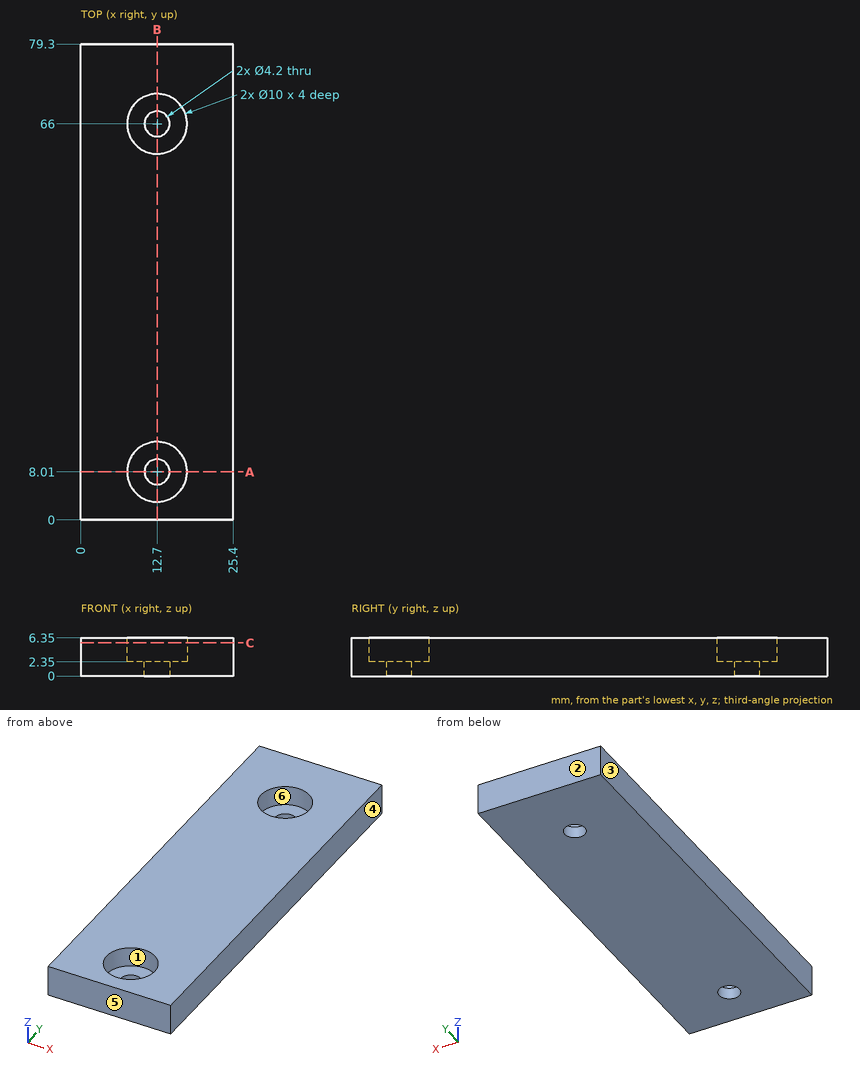
The drawing under review shows one solid part. Ordinate dimensions are in mm from its lowest x, y, z. A direction names the side the tool comes from. Coordinates: 2 decimals unless noted, no trailing zeros. Order: outer loops, then holes, each group sorted by start corner. A loop starts at its lowest first (then second) coordinate and runs counter-clockwise, first axis right, second up. Notation, with made-up numbers: M 64,-18 L 98,-18 A26 ccw 98,4 Z; hole C 30,11 d8. An arc over 180 degrees is marked long. Use a Markdown table: item, result.
(1) Add section B-B (x = 12.7). Give the boundary of the cut face in (y, z).
Worked answers:
| item | result |
|---|---|
| outline | M 0,0 L 5.91,0 L 5.91,2.35 L 3.01,2.35 L 3.01,6.35 L 0,6.35 Z; M 10.11,0 L 63.9,0 L 63.9,2.35 L 61,2.35 L 61,6.35 L 13.01,6.35 L 13.01,2.35 L 10.11,2.35 Z; M 68.1,0 L 79.3,0 L 79.3,6.35 L 71,6.35 L 71,2.35 L 68.1,2.35 Z |
(2) Add section C-C (z = 5.5). Give the boundary of the cut face in (x, y).
Worked answers:
| item | result |
|---|---|
| outline | M 0,0 L 25.4,0 L 25.4,79.3 L 0,79.3 Z; hole C 12.7,8.01 d10; hole C 12.7,66 d10 |
(3) Wall thickness on probe 1 along Y at (x, z) = (12.7, 1.4); probe 2 along Y at (x, z) = (12.7, 4.4); probe 3 along X at (y, z) = (69.5, 5.75): over which ranges is each line inside the solid? List them lowest first.
Worked answers:
| item | result |
|---|---|
| probe 1 | y = 0 to 5.91, 10.11 to 63.9, 68.1 to 79.3 |
| probe 2 | y = 0 to 3.01, 13.01 to 61, 71 to 79.3 |
| probe 3 | x = 0 to 9.13, 16.27 to 25.4 |
(4) For P1, Ø9, axis at x = 12.7, y = 8.01, coming from the +Z side; P2, Ø2.5, axis at x = 12.7, y = 66, coming from the +Z side, all flat-tipped, find the tip position at first contact; note any pin that passes through.
Worked answers:
| item | result |
|---|---|
| P1 | stops at z = 2.35 |
| P2 | passes through |
(5) Draft analysis for pull direction X (two halves, no side actions). For the marked faces 3, 4, 5 and 6, state which applies: released by +X, released by -X, zero draft, split by the parting line, or undercut.
Worked answers:
| item | result |
|---|---|
| face 3 | released by -X |
| face 4 | released by +X |
| face 5 | zero draft |
| face 6 | undercut |
(6) Add section A-A (y = 8.01). Give the boundary of the cut face in (x, z), then the cut area to 3 significant figures.
Worked answers:
| item | result |
|---|---|
| outline | M 0,0 L 10.6,0 L 10.6,2.35 L 7.7,2.35 L 7.7,6.35 L 0,6.35 Z; M 14.8,0 L 25.4,0 L 25.4,6.35 L 17.7,6.35 L 17.7,2.35 L 14.8,2.35 Z |
| area | 111 mm2 |
(7) For the marked faces 1 and 2, list the 3-axis set-ups (+Z, -Z, +X, -X, +Y, -Y) from which the entire face can be reached by the end or side of a thin tool; tool diameter is ignored.
Worked answers:
| item | result |
|---|---|
| face 1 | +Z |
| face 2 | +Z, -Z, +X, -X, +Y |
